Solid Edge part; units mm, degrees
sketch "Sketch1" plane through (0, 0, 0) normal (0, 0, 1) x (1, 0, 0)
  line L0 (49.5, -39) -> (49.5, 39)
  line L1 (49.5, 39) -> (-49.5, 39)
  line L2 (-49.5, 39) -> (-49.5, -39)
  line L3 (-49.5, -39) -> (49.5, -39)
extrude "Protrusion1" add sketch "Sketch1" along normal blind 2.8
sketch "Sketch2" plane through (0, 0, 2.8) normal (0, 0, 1) x (-1, 0, 0)
  line L0 (48.8, -38.3) -> (48.8, 38.3)
  line L1 (48.8, 38.3) -> (-48.8, 38.3)
  line L2 (-48.8, 38.3) -> (-48.8, -38.3)
  line L3 (-48.8, -38.3) -> (48.8, -38.3)
extrude "VaciadoExtruido_1" cut sketch "Sketch2" against normal blind 1.4
sketch "Sketch3" plane through (-49.5, 0, 1.4) normal (-1, 0, 0) x (0, -1, 0)
  line L0 (5.5, 2.8) -> (-5.5, 2.8)
  line L1 (-5.5, 2.8) -> (-5.5, 0)
  line L2 (-5.5, 0) -> (5.5, 0)
  line L3 (5.5, 0) -> (5.5, 2.8)
extrude "VaciadoExtruido_2" cut sketch "Sketch3" against normal blind 100.11
sketch "Sketch4" plane through (0, 0, 1.4) normal (0, 0, 1) x (0, -1, 0)
  circle A0 centre (-25, 42.75) radius 2.4
  circle A1 centre (25, 42.75) radius 2.4
  circle A2 centre (25, -42.75) radius 2.4
  circle A3 centre (-25, -42.75) radius 2.4
extrude "ProtrusiónExtruida_2" add sketch "Sketch4" along normal blind 2.8
sketch "Sketch5" plane through (0, 0, 1.4) normal (0, 0, 1) x (0, -1, 0)
  circle A0 centre (25, 42.75) radius 1.2
  circle A1 centre (-25, 42.75) radius 1.2
  circle A2 centre (-25, -42.75) radius 1.2
  circle A3 centre (25, -42.75) radius 1.2
extrude "VaciadoExtruido_4" cut sketch "Sketch5" along normal blind 2.8
sketch "Sketch6" plane through (0, 0, 1.4) normal (0, 0, 1) x (0, -1, 0)
  line L0 (-19, -47.4) -> (-19, -23.4)
  line L1 (-19, -23.4) -> (-17.6, -23.4)
  line L2 (-17.6, -23.4) -> (-17.6, -47.4)
  line L3 (-17.6, -47.4) -> (-19, -47.4)
  line L4 (-17.6, 23.4) -> (-17.6, 47.4)
  line L5 (-17.6, 47.4) -> (-19, 47.4)
  line L6 (-19, 47.4) -> (-19, 23.4)
  line L7 (-19, 23.4) -> (-17.6, 23.4)
extrude "VaciadoExtruido_5" cut sketch "Sketch6" against normal blind 1
sketch "Sketch7" plane through (0, 0, 0) normal (0, 0, 1) x (1, 0, 0)
  line L0 (-49.5, -39) -> (49.5, -39)
  line L1 (49.5, -39) -> (49.5, 39)
  line L2 (49.5, 39) -> (-49.5, 39)
  line L3 (-49.5, 39) -> (-49.5, -39)
  line L4 (52.1, -41.6) -> (52.1, 41.6)
  line L5 (52.1, 41.6) -> (-52.1, 41.6)
  line L6 (-52.1, 41.6) -> (-52.1, -41.6)
  line L7 (-52.1, -41.6) -> (52.1, -41.6)
extrude "ProtrusiónExtruida_3" add sketch "Sketch7" along normal blind 1.4
sketch "Sketch8" plane through (0, 0, 1.4) normal (0, 0, 1) x (0, 1, 0)
  line L0 (-39, -49.5) -> (-40.4, -49.5)
  line L1 (-40.4, -49.5) -> (-40.4, -48.8)
  line L2 (-40.4, -48.8) -> (-39, -48.8)
  line L3 (-39, -48.8) -> (-39, -49.5)
  line L4 (-41.6, 42.1) -> (-41.6, -42.1)
  line L5 (-41.6, -42.1) -> (-40.2, -42.1)
  line L6 (-40.2, -42.1) -> (-40.2, 42.1)
  line L7 (-40.2, 42.1) -> (-41.6, 42.1)
  line L8 (-40.4, 48.8) -> (-39, 48.8)
  line L9 (-39, 48.8) -> (-39, 49.5)
  line L10 (-39, 49.5) -> (-40.4, 49.5)
  line L11 (-40.4, 49.5) -> (-40.4, 48.8)
  line L12 (40.4, 48.8) -> (39, 48.8)
  line L13 (39, 48.8) -> (39, 49.5)
  line L14 (39, 49.5) -> (40.4, 49.5)
  line L15 (40.4, 49.5) -> (40.4, 48.8)
  line L16 (40.2, -42.1) -> (40.2, 42.1)
  line L17 (40.2, 42.1) -> (41.6, 42.1)
  line L18 (41.6, 42.1) -> (41.6, -42.1)
  line L19 (41.6, -42.1) -> (40.2, -42.1)
  line L20 (39, -49.5) -> (40.4, -49.5)
  line L21 (40.4, -49.5) -> (40.4, -48.8)
  line L22 (40.4, -48.8) -> (39, -48.8)
  line L23 (39, -48.8) -> (39, -49.5)
extrude "ProtrusiónExtruida_4" add sketch "Sketch8" along normal blind 1.4
Work out the finished part from the listing and answer in its coordinate system (mm). A direction names the side the tool comes from. Give positions to 0.01 mm unless a question says otherwise; leave off trailing zeros. Order: outer loops, then holes, each group sorted by start corner. A loop starts at its lowest first (then second) coordinate and runs counter-clockwise, first axis right, second up. Notation, with made-up numbers: (62.5, 45) - (100.5, 45) arc R17 cw to (100.5, 50) - close; hole circle Ø3 at (47.5, 74). An arc over 180 degrees is marked (long way). Answer as CSV lines item,"result". Start each with the question number.
Q1. The part is cut by section C-C (x = 37). Write down the section's boundary in (y, z).
Q2. The part is cut by section A-A (y = -20). Write down the section's boundary in (x, z), then the cut area to 3 significant figures.
Q3. Given pin 1 Ø1.5 at (y, z) = (18, 2) entering from -X; pin 2 Ø0.7 at (y, z) = (16.5, 2) entering from +X; pin 3 Ø0.6 at (x, z) = (49.5, 2) entering from -Y; pin 4 Ø2 at (x, y) = (-32, -27) entering from +Z, each flat-ended and moving along its own axis, determine where each tip first touches the part or whether it passes through.
Q4. The mould has two halves that part along Y. Classify faces 1 (the face through (-1, 1, 0)), 2 (the face through (1, 41.6, 1)), 3 (the face through (43, -25, 1.4)): +Y half, -Y half, draft (parallel to the pull), parting line (faces both ways), or undercut.
Q5. The part is cut by section D-D (y = -2.5). Write down the section's boundary in (x, z), then the cut area to 3 significant figures.
Q6. For faces 4 (the face through (-44, -24, 4.2)), 5 (the face through (-43.94, -24.84, 2.78)), determine the directions among +Z, -Z, +X, -X, +Y, -Y from which every point of the face is accessible in a straight line to the end or side of a thin tool.
Q7. The part is cut by section B-B (x = 10.5). Write down the section's boundary in (y, z), then the cut area to 3 significant figures.
Q8. Find the intervals of material crossed by L1, parallel to Y at x = -29.5, z = 2.25; L2, parallel to X at y = -25, z = 2.4; L3, parallel to X at y = 25, z = 3.35, in increasing order. Write a range as [from, to].
Check result:
1,outline,"(-41.6, 0) - (41.6, 0) - (41.6, 2.8) - (40.2, 2.8) - (40.2, 1.4) - (39, 1.4) - (39, 2.8) - (38.3, 2.8) - (38.3, 1.4) - (19, 1.4) - (19, 0.4) - (17.6, 0.4) - (17.6, 1.4) - (-38.3, 1.4) - (-38.3, 2.8) - (-39, 2.8) - (-39, 1.4) - (-40.2, 1.4) - (-40.2, 2.8) - (-41.6, 2.8) - close"
2,outline,"(-52.1, 0) - (52.1, 0) - (52.1, 1.4) - (49.5, 1.4) - (49.5, 2.8) - (48.8, 2.8) - (48.8, 1.4) - (-48.8, 1.4) - (-48.8, 2.8) - (-49.5, 2.8) - (-49.5, 1.4) - (-52.1, 1.4) - close"
2,area,"148 mm²"
3,pin 1,"stops at x = -52.1"
3,pin 2,"stops at x = 49.5"
3,pin 3,"stops at y = -40.4"
3,pin 4,"stops at z = 1.4"
4,face 1,"draft"
4,face 2,"+Y half"
4,face 3,"undercut"
5,outline,"(-52.1, 0) - (52.1, 0) - (52.1, 1.4) - (-52.1, 1.4) - close"
5,area,"146 mm²"
6,face 4,"+Z, +X, -X, +Y, -Y"
6,face 5,"+Z"
7,outline,"(-41.6, 0) - (41.6, 0) - (41.6, 2.8) - (40.2, 2.8) - (40.2, 1.4) - (39, 1.4) - (39, 2.8) - (38.3, 2.8) - (38.3, 1.4) - (-38.3, 1.4) - (-38.3, 2.8) - (-39, 2.8) - (-39, 1.4) - (-40.2, 1.4) - (-40.2, 2.8) - (-41.6, 2.8) - close"
7,area,"122 mm²"
8,L1,"y = [-41.6, -40.2], [-39, -38.3], [38.3, 39], [40.2, 41.6]"
8,L2,"x = [-49.5, -48.8], [-45.15, -43.95], [-41.55, -40.35], [40.35, 41.55], [43.95, 45.15], [48.8, 49.5]"
8,L3,"x = [-45.15, -43.95], [-41.55, -40.35], [40.35, 41.55], [43.95, 45.15]"
